from build123d import *

# Parameters (mm, degrees)
SKETCH1_W           = 20
SKETCH1_H           = 80
SKETCH1_R           = 5
BOSS_EXTRUDE1_DEPTH = 5
BOSS_EXTRUDE2_DEPTH = 7.5
BOSS_EXTRUDE3_DEPTH = 5
SKETCH4_R           = 5
BOSS_EXTRUDE4_DEPTH = 105


with BuildPart() as part:
    # Sketch1 → Boss-Extrude1 (new, symmetric)
    with BuildSketch(Plane.XY):
        with Locations((0, 40)):
            Rectangle(SKETCH1_W, SKETCH1_H)
        with Locations((0, 12)):
            Circle(SKETCH1_R, mode=Mode.SUBTRACT)
    extrude(amount=BOSS_EXTRUDE1_DEPTH, both=True)

    # Sketch2 → Boss-Extrude2 (add, symmetric)
    with BuildSketch(Plane.XY):
        Polygon((-15, 80), (-15, 170), (5, 200), (25, 200), (25, 187.5), (12.5, 175), (25, 162.5), (25, 150), (15, 150), (15, 80), align=None)
    extrude(amount=BOSS_EXTRUDE2_DEPTH, both=True)

    # Sketch3 → Boss-Extrude3 (add, symmetric)
    with BuildSketch(Plane.XY):
        with BuildLine():
            Line((-7.071067812, 19.071067812), (-28.284271247, -2.142135624))
            Line((-28.284271247, -2.142135624), (-14.142135624, -16.284271247))
            Line((-14.142135624, -16.284271247), (7.071067812, 4.928932188))
            Line((7.071067812, 4.928932188), (3.535533906, 8.464466094))
            ThreePointArc((3.535533906, 8.464466094), (-3.535533906, 8.464466094), (-3.535533906, 15.535533906))
            Line((-3.535533906, 15.535533906), (-7.071067812, 19.071067812))
        make_face()
    extrude(amount=BOSS_EXTRUDE3_DEPTH, both=True)

    # Sketch4 → Boss-Extrude4 (add)
    with BuildSketch(Plane(origin=(-15.213203436, -15.213203436, 0), x_dir=(0, 0, 1), z_dir=(-0.7071067811865512, -0.7071067811865438, 0))):
        with Locations(Location((0, 8.485281374, 0), (0, 0, 180))):
            Circle(SKETCH4_R)
    extrude(amount=BOSS_EXTRUDE4_DEPTH)


solid = part.part
Model file for the job. Use its own axes, mm. A direction names the side the tool comes from. Round coordinates to 2 decimals unless told otherwise and drop trailing zeros. Loops run counter-clockwise (first coordinate to the right, second up) from the corner with the lowest first, then second, coordinate; pieces in that order, holes last. Notation, with made-up numbers: (77.5, 21.5) -> (94.5, 21.5) arc R30 ccw to (94.5, 44.5) -> close; hole circle Ø8 at (-1, 25). An arc over 180 degrees is marked (long way). Answer as CSV lines item,"result". Start each with the question number.
1) Slice it at A-A (z = -2). List the corners of the cut face in (x, y).
2) Slice it at C-C (y = 77). List the corners of the cut face in (x, z).
3) Pin check, flat tips, straight feed: P1, Ø3, axis at y = 43.5, z = -2, coming from the -X side; P2, Ø5, axis at y = 33, z = 1.5, coming from the +X side; P3, Ø5, axis at x = 18, z = 1.5, coming from the -Y side. Stop position of each tip, or through.
4) Mould opens along X. For faces 1 (the face through (6, 0, 0)), 2 (the face through (-26.37, -4.057, 0.07)), 3 (the face through (-16.156, -14.271, 0.07)) say: +X half, -X half, draft (parallel to the pull), parting line (faces both ways), or undercut.
5) Tool access for faces 4 (the face through (18.8, 181.3, 0.1)), 5 (the face through (20, 150, 0)), 6 (the face through (-19.01, 7.13, 0.07)), 7 (the face through (-15, 124, 0)), 8 (the face through (0, 80, 7)): list every direction of +Z, -Z, +X, -X, +Y, -Y with a clear straight run to the whole face (end or side of a thin tool).
6) Slice it at B-B (y = 132.5). List the corners of the cut face in (x, z), plus the area to 3 significant figures.
7) Probe line 1 along X through (y, z) = (122.5, 4.5); line 2 along X through (y, z) = (158.5, 0.5); line 3 along Z through (x, y) = (3.5, 36). List the from-to ranges inside material, lowest first.
Filled in:
1,outline,"(-98.7, -80.22) -> (-92.22, -86.7) -> (-17.97, -12.45) -> (-14.14, -16.28) -> (2.14, 0) -> (10, 0) -> (10, 80) -> (15, 80) -> (15, 150) -> (25, 150) -> (25, 162.5) -> (12.5, 175) -> (25, 187.5) -> (25, 200) -> (5, 200) -> (-15, 170) -> (-15, 80) -> (-10, 80) -> (-10, 16.14) -> (-28.28, -2.14) -> (-24.45, -5.97) -> close; hole circle Ø10 at (0, 12)"
2,outline,"(-10, -5) -> (10, -5) -> (10, 5) -> (-10, 5) -> close"
3,P1,"stops at x = -10"
3,P2,"stops at x = 10"
3,P3,"stops at y = 150"
4,face 1,"draft"
4,face 2,"-X half"
4,face 3,"undercut"
5,face 4,"+Z, -Z, +X"
5,face 5,"+Z, -Z, +X, -Y"
5,face 6,"+Z, -Z, -X"
5,face 7,"+Z, -Z, -X, +Y"
5,face 8,"none"
6,outline,"(-15, -7.5) -> (15, -7.5) -> (15, 7.5) -> (-15, 7.5) -> close"
6,area,"450 mm2"
7,line 1,"x = -15 to 15"
7,line 2,"x = -15 to 25"
7,line 3,"z = -5 to 5"
